```python
from build123d import *

# Parameters (mm, degrees)
SKETCH1_W           = 130
SKETCH1_H           = 80
BOSS_EXTRUDE1_DEPTH = 2.8
SKETCH2_W           = 14.444444444
SKETCH2_H           = 2.8
SKETCH2_W_2         = 2.8
SKETCH2_H_2         = 13.333333334
SKETCH2_H_3         = 13.333333333
CUT_EXTRUDE1_DEPTH  = 153.669053839
CUT_EXTRUDE2_REACH  = 154.669
SKETCH3_R           = 1.7


with BuildPart() as part:
    # Sketch1 → Boss-Extrude1 (new body)
    with BuildSketch(Plane.XY):
        with Locations((65, 40)):
            Rectangle(SKETCH1_W, SKETCH1_H)
    extrude(amount=BOSS_EXTRUDE1_DEPTH)

    # Sketch2 → Cut-Extrude1 (cut, through all)
    with BuildSketch(Plane.XY.offset(2.8)):
        with Locations((7.222222222, 1.4)):
            Rectangle(SKETCH2_W, SKETCH2_H)
        with Locations((36.111111111, 1.4)):
            Rectangle(SKETCH2_W, SKETCH2_H)
        with Locations((65, 1.4)):
            Rectangle(SKETCH2_W, SKETCH2_H)
        with Locations((93.888888889, 1.4)):
            Rectangle(SKETCH2_W, SKETCH2_H)
        Polygon((115.555555556, 0), (115.555555556, 2.8), (127.2, 2.8), (127.2, 13.333333333), (130, 13.333333333), (130, 0), align=None)
        with Locations((1.4, 20)):
            Rectangle(SKETCH2_W_2, SKETCH2_H_2)
        with Locations((1.4, 46.666666667)):
            Rectangle(SKETCH2_W_2, SKETCH2_H_3)
        with Locations((1.4, 73.333333334)):
            Rectangle(SKETCH2_W_2, SKETCH2_H_3)
        with Locations((128.6, 33.333333334)):
            Rectangle(SKETCH2_W_2, SKETCH2_H_3)
        with Locations((128.6, 60)):
            Rectangle(SKETCH2_W_2, SKETCH2_H_2)
    extrude(amount=-CUT_EXTRUDE1_DEPTH, mode=Mode.SUBTRACT)

    # Sketch3 → Cut-Extrude2 (cut, up to next)
    with BuildSketch(Plane.XY.offset(2.8), mode=Mode.PRIVATE) as cut_extrude2_sk1:
        with Locations((14.8, 74.5)):
            Circle(SKETCH3_R)
    cut_extrude2_tool1 = extrude(cut_extrude2_sk1.sketch, amount=-CUT_EXTRUDE2_REACH, mode=Mode.PRIVATE) & part.part
    # Sketch3 → Cut-Extrude2 (cut, up to next)
    with BuildSketch(Plane.XY.offset(2.8), mode=Mode.PRIVATE) as cut_extrude2_sk2:
        with Locations(Location((115.2, 74.5, 0), (0, 0, 180))):
            Circle(SKETCH3_R)
    cut_extrude2_tool2 = extrude(cut_extrude2_sk2.sketch, amount=-CUT_EXTRUDE2_REACH, mode=Mode.PRIVATE) & part.part
    # Sketch3 → Cut-Extrude2 (cut, up to next)
    with BuildSketch(Plane.XY.offset(2.8), mode=Mode.PRIVATE) as cut_extrude2_sk3:
        with Locations((14.8, 11.124824394)):
            Circle(SKETCH3_R)
    cut_extrude2_tool3 = extrude(cut_extrude2_sk3.sketch, amount=-CUT_EXTRUDE2_REACH, mode=Mode.PRIVATE) & part.part
    # Sketch3 → Cut-Extrude2 (cut, up to next)
    with BuildSketch(Plane.XY.offset(2.8), mode=Mode.PRIVATE) as cut_extrude2_sk4:
        with Locations((115.2, 11.124824394)):
            Circle(SKETCH3_R)
    cut_extrude2_tool4 = extrude(cut_extrude2_sk4.sketch, amount=-CUT_EXTRUDE2_REACH, mode=Mode.PRIVATE) & part.part
    add(cut_extrude2_tool1.solids().sort_by_distance((14.8, 74.5, 2.8))[0], mode=Mode.SUBTRACT)
    add(cut_extrude2_tool2.solids().sort_by_distance((115.2, 74.5, 2.8))[0], mode=Mode.SUBTRACT)
    add(cut_extrude2_tool3.solids().sort_by_distance((14.8, 11.124824, 2.8))[0], mode=Mode.SUBTRACT)
    add(cut_extrude2_tool4.solids().sort_by_distance((115.2, 11.124824, 2.8))[0], mode=Mode.SUBTRACT)


solid = part.part
```
CAD build for the part. Positions are in the model's coordinates, mm. A direction names the side the tool comes from. Coordinates: 2 decimals unless noted, no trailing zeros. Order: outer loops, then holes, each group sorted by start corner. A loop starts at its lowest first (then second) coordinate and runs counter-clockwise, first axis right, second up. Notation, with made-up numbers: M 35.25,36.25 L 94.25,36.25 A8 ccw 94.25,40.25 Z; hole C 4,82.5 d4. An arc over 180 degrees is marked long. Write each question's results on one line, items separated by ' | '. Start each with the question number.
Q1. Which spindle directions (+Z, -Z, +X, -X, +Y, -Y) get a long thin tool onto all of the face, cutting with end or side? Do faces 1 (the flat face through (101.111, 1, 1)), 2 (the flat face through (7, 2.8, 1)), 3 (the flat face through (1, 53.333, 1)). Say none if no direction does.
Q2. Drill centre lines: probe 1 along Y at (x, z) = (14.8, 0.6); probe 2 along X at (y, z) = (74.5, 0.85); probe 3 along X at (y, z) = (73, 2.55). Where is each one in solid material? Low to high. Write a range as from..to.
Q3. Flat gauge pins, fed straight in: P1, Ø1.4, axis at y = 6, z = 2, coming from the +X side; P2, Ø0.8, axis at x = 90.5, z = 2, coming from the -Y side; P3, Ø1.4, axis at x = 128.5, z = 2, coming from the -Y side; P4, Ø1.5, axis at x = 23.5, z = 1.5, coming from the -Y side. Where does each tip first touch, or does it go through?
Q4. Cut at A-A (y = 74.5). List the corners of the cut face in (x, z), then the cut area to 3 significant figures.
Q5. Cut at D-D (y = 37). List the corners of the cut face in (x, z).
Q6. Cut at C-C (z = 1.9). Count the separate pieces of the cut face and the enclosed holes in it, then the cut area to 3 significant figures.
Q7. Cut at B-B (x = 63). List the corners of the cut face in (y, z), then the cut area to 3 significant figures.
Q8. Pull direction X, two halves, no side cores. Call faces 4 (the flat face through (0, 60, 1)), 5 (the flat face through (108, 0, 1)), 6 (the flat face through (43.333, 1, 1)): +X half, -X half, draft (parallel to the pull), parting line (faces both ways), or undercut.
Found:
1) face 1: +Z, -Z, -Y | face 2: +Z, -Z, -X, -Y | face 3: +Z, -Z, -X
2) probe 1: 0..9.42, 12.82..72.8, 76.2..80 | probe 2: 2.8..13.1, 16.5..113.5, 116.9..130 | probe 3: 2.8..14, 15.6..114.4, 116..130
3) P1: x = 127.2 | P2: y = 2.8 | P3: y = 13.33 | P4: y = 0
4) outline: M 2.8,0 L 13.1,0 L 13.1,2.8 L 2.8,2.8 Z; M 16.5,0 L 113.5,0 L 113.5,2.8 L 16.5,2.8 Z; M 116.9,0 L 130,0 L 130,2.8 L 116.9,2.8 Z | area: 337 mm²
5) outline: M 0,0 L 127.2,0 L 127.2,2.8 L 0,2.8 Z
6) separate pieces: 1 | enclosed holes: 4 | area: 9,950 mm²
7) outline: M 2.8,0 L 80,0 L 80,2.8 L 2.8,2.8 Z | area: 216 mm²
8) face 4: -X half | face 5: draft | face 6: undercut
